```python
from build123d import *

# Parameters (mm, degrees)
SKETCH1_R           = 0.875
BOSS_EXTRUDE1_DEPTH = 7
SKETCH2_R           = 1.625
BOSS_EXTRUDE2_DEPTH = 1.5
FILLET1_R           = 0.15
CHAMFER1_SIZE       = 0.15
CUT_EXTRUDE1_DEPTH  = 0.8
CHAMFER2_SIZE       = 0.075
FILLET2_R           = 0.075


with BuildPart() as part:
    # Sketch1 → Boss-Extrude1 (new body)
    with BuildSketch(Plane(origin=(0, 0, 0), x_dir=(1, 0, 0), z_dir=(0, 1, 0))):
        with Locations(Location((0, 0, 0), (0, 0, 270))):
            Circle(SKETCH1_R)
    extrude(amount=BOSS_EXTRUDE1_DEPTH)

    # Sketch2 → Boss-Extrude2 (add)
    with BuildSketch(Plane(origin=(0, 7, 0), x_dir=(1, 0, 0), z_dir=(0, 1, 0))):
        with Locations(Location((0, 0, 0), (0, 0, 270))):
            Circle(SKETCH2_R)
    extrude(amount=BOSS_EXTRUDE2_DEPTH)

    # Fillet1
    fillet1_edges = [part.edges().sort_by_distance(p)[0] for p in [
        (0, 7, -0.875),
    ]]
    fillet(fillet1_edges, radius=FILLET1_R)

    # Chamfer1
    chamfer1_edges = [part.edges().sort_by_distance(p)[0] for p in [
        (0, 7, -1.625),
        (0, 8.5, -1.625),
    ]]
    chamfer(chamfer1_edges, length=CHAMFER1_SIZE)

    # Sketch3 → Cut-Extrude1 (cut)
    with BuildSketch(Plane(origin=(0, 8.5, 0), x_dir=(1, 0, 0), z_dir=(0, 1, 0))):
        Polygon((0, 1.010362971), (-0.875, 0.505181486), (-0.875, -0.505181486), (0, -1.010362971), (0.875, -0.505181486), (0.875, 0.505181486), align=None)
    extrude(amount=-CUT_EXTRUDE1_DEPTH, mode=Mode.SUBTRACT)

    # Chamfer2
    chamfer2_edges = [part.edges().sort_by_distance(p)[0] for p in [
        (0, 0, -0.875),
    ]]
    chamfer(chamfer2_edges, length=CHAMFER2_SIZE)

    # Fillet2
    fillet2_edges = [part.edges().sort_by_distance(p)[0] for p in [
        (0.4375, 7.7, -0.757772228),
        (0, 8.1, -1.010362971),
        (0.875, 7.7, 0),
        (0.875, 8.1, -0.505181486),
        (0.4375, 7.7, 0.757772228),
        (0.875, 8.1, 0.505181486),
        (-0.4375, 7.7, 0.757772228),
        (0, 8.1, 1.010362971),
        (-0.875, 7.7, 0),
        (-0.875, 8.1, 0.505181486),
        (-0.4375, 7.7, -0.757772228),
        (-0.875, 8.1, -0.505181486),
        (0.4375, 8.5, -0.757772228),
        (-0.4375, 8.5, -0.757772228),
        (-0.875, 8.5, 0),
        (-0.4375, 8.5, 0.757772228),
        (0.4375, 8.5, 0.757772228),
        (0.875, 8.5, 0),
    ]]
    fillet(fillet2_edges, radius=FILLET2_R)


solid = part.part
```
Part model, mm, in its own coordinate system. Round coordinates to 2 decimals unless told otherwise and drop trailing zeros. Order: outer loops, then holes, each group sorted by start corner. A loop starts at its lowest first (then second) coordinate and runs counter-clockwise, first axis right, second up. Notation, with made-up numbers: M -9,37.5 L 24,37.5 A11 cw 24,54.5 Z; hole C -35.5,9.5 d8. An arc over 180 degrees is marked long. Answer in a Markdown table with one row per item. Add a question column.
Q1. Cut at A-A on z = 0. Give the cut face in (x, y) (3 decimals).
Q2. Mould opens along X. For faces 1 (the face through (0, 7.7, 0)), 2 (the face through (0, 0, 0)), 3 (the face through (-0.854, 3.415, -0.19)) say: +X half, -X half, draft (parallel to the pull), parting line (faces both ways), or undercut.
Q3. Cut at B-B on y = 2.5. Give the cut face in (x, z) (3 decimals), and give its area (3 significant figures).
Q4. Pin check, flat tip, straight feed: pin 1 (0.5 mm diameter, centred on x = -0.5, z = 0, fed in from +Y). Stop position of the tip, or through.
Q5. Cut at C-C on y = 7.5. Give the cut face in (x, z) (3 decimals).
Q6. Wall check: L1, parallel to X at y = 8, z = -0.3 (3 decimals); L2, parallel to Y at x = 0.35, z = -1.05; L3, parallel to Y at x = -0.3, z = 0.2. Give the ranges that are in metal, low to high. Write a range as from..to.
Established:
| question | item | result |
|---|---|---|
| 1 | outline | M -1.625,7.15 L -1.475,7 L -1.025,7 A0.15 cw -0.875,6.85 L -0.875,0.075 L -0.8,0 L 0.8,0 L 0.875,0.075 L 0.875,6.85 A0.15 cw 1.025,7 L 1.475,7 L 1.625,7.15 L 1.625,8.35 L 1.475,8.5 L 0.95,8.5 A0.075 ccw 0.875,8.425 L 0.875,7.775 A0.075 cw 0.8,7.7 L -0.8,7.7 A0.075 cw -0.875,7.775 L -0.875,8.425 A0.075 ccw -0.95,8.5 L -1.475,8.5 L -1.625,8.35 Z |
| 2 | face 1 | undercut |
| 2 | face 2 | draft |
| 2 | face 3 | parting line |
| 3 | outline | C 0,0 d1.75 |
| 3 | area | 2.41 mm2 |
| 4 | pin 1 | stops at y = 7.7 |
| 5 | outline | C 0,0 d3.25 |
| 6 | L1 | x = -1.597..-0.875, 0.875..1.597 |
| 6 | L2 | y = 7..8.5 |
| 6 | L3 | y = 0..7.7 |
